Here's how the part is built. I have some questions about the finished solid (model axes, mm). Face numbers are marked on the shaded views. A direction names the side the tool comes from. Coordinates: 2 decimals unless noted, no trailing zeros. Loops run counter-clockwise (first coordinate to the right, second up) from the corner with the lowest first, then second, coordinate; pieces in that order, holes last. Notation, with made-up numbers: (68.25, 40) -> (75.25, 40) arc R35 cw to (75.25, 73) -> close; hole circle Ø9 at (83.5, 7). An arc over 180 degrees is marked (long way). Answer as a JSON object with one key per item and string values. Group by question number.
Q1. I want a section at A-A on y = 5. Count the separate pieces of the cut face and the enclosed holes in it, then the cut area to 3 significant figures.
Q2. I'm going to push flat-ended pins straight in: pin 1 (1 mm diameter, centred on y = 1, z = 37, fed in from +X); pin 2 (1 mm diameter, centred on x = 57, y = 4.5, fed in from -Z); pin 3 (1.6 mm diameter, centred on x = 19.05, z = 75, fed in from -Y); pin 4 (1.5 mm diameter, centred on x = 25, y = 2.5, fed in from -Z). Where does each tip first touch, or does it pass through?
Q3. I need wall thicknesses on line 1 (X direction, y = 4.5, z = 0); line 2 (X direction, y = 1.75, z = -75); line 3 (Z direction, x = -19.05, y = 1.5). Which ranges of each line are inside material? Lowest first, please.
Q4. Thinking about a two-plate mould opening in X: for the marked faces 3 and 4, which applies, released by +X, released by -X, zero draft, split by the parting line, or undercut?
Q5. On a 3-axis mill with a long thin cutter (end or side, diameter ignored), from which of +Z, -Z, +X, -X, +Y, -Y can I reach the whole of each face in a straight line? I mean the marked faces 1 and 2. Say none if no direction works.
Q6. I want a section at B-B on x = -52.5. Write out the boundary of the cut face in (y, z).
Q7. I want a section at C-C on z = 53. Write out the boundary of the cut face in (x, y).
```python
from build123d import *

# Parameters (mm, degrees)
SKETCH2_R             = 93.485122645
EXTRUDE1_DEPTH        = 7
SKETCH3_R             = 8
CUT_EXTRUDE1_DEPTH    = 8
F_3_48_TAPPED_HOLE1_D = 1.9939
CIRPATTERN1_COUNT     = 4
SKETCH8_R             = 60
CUT_EXTRUDE2_DEPTH    = 8
SKETCH9_R             = 60
CUT_EXTRUDE10_DEPTH   = 4
CIRPATTERN4_COUNT     = 4


with BuildPart() as part:
    # Sketch2 → Extrude1 (new body)
    with BuildSketch(Plane(origin=(0, 0, 0), x_dir=(1, 0, 0), z_dir=(0, 1, 0))):
        Circle(SKETCH2_R)
    extrude(amount=EXTRUDE1_DEPTH)

    # Sketch3 → Cut-Extrude1 (cut, through all)
    with BuildSketch(Plane(origin=(0, 7, 0), x_dir=(1, 0, 0), z_dir=(0, 1, 0))):
        with Locations((0, 75)):
            Circle(SKETCH3_R)
    cut_extrude1 = extrude(amount=-CUT_EXTRUDE1_DEPTH, mode=Mode.SUBTRACT)

    # #3-48 Tapped Hole1 (through all)
    with Locations(Plane(origin=(0, 7, 0), x_dir=(1, 0, 0), z_dir=(0, 1, 0))):
        with Locations((-19.05, 75), (19.05, 75)):
            f_3_48_tapped_hole1 = Hole(F_3_48_TAPPED_HOLE1_D / 2)

    # CirPattern1: Cut-Extrude1, #3-48 Tapped Hole1 ×4 about axis
    cirpattern1_axis = Axis((0, 0, 0), (0, 1, 0))
    for i in range(1, CIRPATTERN1_COUNT):
        add(cut_extrude1.rotate(cirpattern1_axis, i * 360 / CIRPATTERN1_COUNT), mode=Mode.SUBTRACT)
        add(f_3_48_tapped_hole1.rotate(cirpattern1_axis, i * 360 / CIRPATTERN1_COUNT), mode=Mode.SUBTRACT)

    # Sketch8 → Cut-Extrude2 (cut, through all)
    with BuildSketch(Plane(origin=(0, 7, 0), x_dir=(1, 0, 0), z_dir=(0, 1, 0))):
        Circle(SKETCH8_R)
    extrude(amount=-CUT_EXTRUDE2_DEPTH, mode=Mode.SUBTRACT)

    # Sketch9 → Cut-Extrude10 (cut)
    with BuildSketch(Plane(origin=(0, 7, 0), x_dir=(1, 0, 0), z_dir=(0, 1, 0))):
        Circle(SKETCH9_R)
        Polygon((41.044204571, -83.470611442), (83.470611442, -41.044204571), (42.459618294, -0.033211423), (-0.033211423, -42.393195448), align=None)
    cut_extrude10 = extrude(amount=-CUT_EXTRUDE10_DEPTH, mode=Mode.SUBTRACT)

    # CirPattern4: Cut-Extrude10 ×4 about axis
    cirpattern4_axis = Axis((0, 0, 0), (0, 1, 0))
    for i in range(1, CIRPATTERN4_COUNT):
        add(cut_extrude10.rotate(cirpattern4_axis, i * 360 / CIRPATTERN4_COUNT), mode=Mode.SUBTRACT)


solid = part.part
```
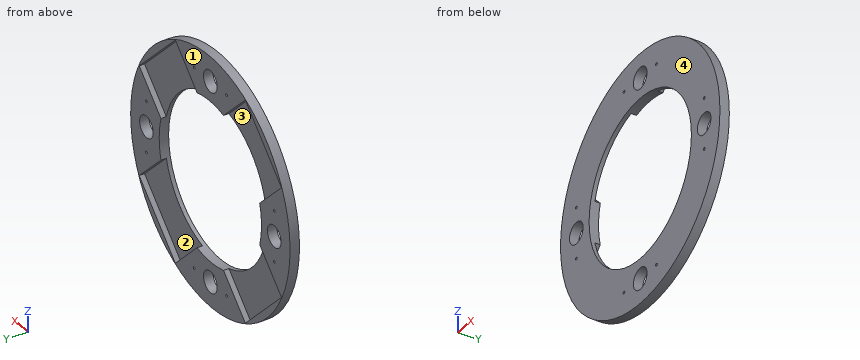
Result set:
{
 "1": {"separate pieces": "1", "enclosed holes": "13", "area": "7,960 mm²"},
 "2": {"pin 1": "stops at x = 86.07", "pin 2": "stops at z = -74.48", "pin 3": "passes through", "pin 4": "stops at z = -90.29"},
 "3": {"line 1": "x = -93.49 to -83, -67 to -60, 60 to 67, 83 to 93.49", "line 2": "x = -55.81 to -20.05, -18.05 to -8, 8 to 18.05, 20.05 to 55.81", "line 3": "z = -91.52 to -76, -74 to -56.9, 56.9 to 74, 76 to 91.52"},
 "4": {"face 3": "undercut", "face 4": "zero draft"},
 "5": {"face 1": "+Z, -Z, +X, -X, +Y", "face 2": "+Y"},
 "6": {"outline": "(0, -77.35) -> (7, -77.35) -> (7, -72.01) -> (3, -72.01) -> (3, -29.05) -> (0, -29.05) -> close; (0, 29.05) -> (3, 29.05) -> (3, 72.01) -> (7, 72.01) -> (7, 77.35) -> (0, 77.35) -> close"},
 "7": {"outline": "(-77.01, 0) -> (-28.12, 0) -> (-28.12, 3) -> (-71.51, 3) -> (-71.51, 7) -> (-77.01, 7) -> close; (28.12, 0) -> (77.01, 0) -> (77.01, 7) -> (71.51, 7) -> (71.51, 3) -> (28.12, 3) -> close"}
}
